```python
from build123d import *

# Parameters (mm, degrees)
F1_DEPTH  = 55
F3_DEPTH  = 50
F4_W      = 46.6654431075
F4_H      = 57.836631313
F5_DEPTH  = 25
F6_R      = 5
F8_D      = 5
F10_DEPTH = 5
F12_DEPTH = 2


with BuildPart() as f1:
    # F0 (on Top) → F1 (new body)
    with BuildSketch(Plane.XY):
        with BuildLine():
            ThreePointArc((0, -20.5), (14.4956890143, -14.4956890143), (20.5, 0))
            ThreePointArc((20.5, 0), (14.4956890143, 14.4956890143), (0, 20.5))
            ThreePointArc((0, 20.5), (-20.5, 0), (0, -20.5))
        make_face()
        with BuildLine():
            ThreePointArc((19, 0), (-13.4350288425, -13.4350288425), (0, 19))
            ThreePointArc((0, 19), (13.4350288425, 13.4350288425), (19, 0))
        make_face(mode=Mode.SUBTRACT)
        with BuildLine():
            ThreePointArc((0, -20.5), (-20.5, 0), (0, 20.5))
            Line((0, 20.5), (-70, 20.5))
            Line((-70, 20.5), (-90, -20.5))
            Line((-90, -20.5), (0, -20.5))
        make_face()
    extrude(amount=F1_DEPTH)

    # F2 (on face) → F3 (cut)
    with BuildSketch(Plane.XY):
        Polygon((-20.693905686, 24.13287099), (-92.3021333856, 24.13287099), (-92.6832251204, -12.49999901), (-75, -15.5), (-75, -22.0035649836), (-20.7452352142, -22.0035649836), align=None)
    extrude(amount=F3_DEPTH, mode=Mode.SUBTRACT)

    # F4 (on face) → F5 (cut)
    with BuildSketch(Plane.XY):
        with Locations((-0.7558101788, 1.7380928621)):
            Rectangle(F4_W, F4_H)
    extrude(amount=F5_DEPTH, mode=Mode.SUBTRACT)

    # F6
    f6_edges = [f1.edges().sort_by_distance(p)[0] for p in [
        (-20.697947, 20.5, 37.5),
        (-20.743562, -20.5, 37.5),
    ]]
    fillet(f6_edges, radius=F6_R)

    # F8 (through all)
    with Locations(Plane.XZ.offset(20.5)):
        with Locations((-80.5, 41.5), (-80.5, 11.5)):
            Hole(F8_D / 2)

    # F9 (on face) → F10 (join)
    with BuildSketch(Plane.XZ.offset(20.5)):
        Polygon((-66.2546011695, 50), (-75, 41.8011878794), (-75, 36.4798588918), (-60.5785174124, 50), align=None)
    extrude(amount=-F10_DEPTH)

    # F11 (on face) → F12 (join)
    with BuildSketch(Plane(origin=(-64.6227775108, 31.5233061028, 0), x_dir=(-0.438423632, -0.8987684456, 0), z_dir=(-0.8987684456, 0.438423632, 0))):
        Polygon((50.1299122344, 50), (38.5309847388, 50), (50.1299122344, 38.7167511187), align=None)
    extrude(amount=-F12_DEPTH)


solid = f1.part
```
Here's how the part is built. I have some questions about the finished solid (model axes, mm). A direction names the side the tool comes from. Give positions to 0.01 mm unless a question says otherwise; leave off trailing zeros. Loops run counter-clockwise (first coordinate to the right, second up) from the corner with the lowest first, then second, coordinate; pieces in that order, holes last. Notation, with made-up numbers: (-8, 43.5) -> (-3, 43.5) arc R6 ccw to (-3, 53.5) -> close; hole circle Ø3 at (66, 34). An arc over 180 degrees is marked (long way). Use one line per item in the form item = value. Start each with the question number.
1) Thinking about a two-plate mould opening in X: for faces 1 (the face through (-69, -15.5, 45)), 2 (the face through (-14, 20.5, 43)), 3 (the face through (-80.9, -14.5, 24.6)), 4 (the face through (-86.62, -13.57, 39.85)), which applies, +X half, -X half, draft (parallel to the pull), parting line (faces both ways), or undercut?
2) Imagine slicing it at C-C (z = 11.5). Please give me the cut outline in (x, y).
3) For P1, Ø4, axis at x = -80.5, z = 11.5, coming from the +Y side; P2, Ø12, axis at y = 5, z = 35, coming from the +X side; P3, Ø1.5, axis at y = -17.5, z = 18, coming from the +X side; P4, Ø11, axis at x = -66, z = 43.5, coming from the +Y side, each with a flat end and sliding along its axis, tell me the tip position at first contact or that it passes through.
4) Imagine slicing it at A-A (z = 32). Please give me the cut outline in (x, y).
5) Imagine slicing it at B-B (y = 14). Please give me the cut outline in (x, z).
6) Which directions (+Z, -Z, +X, -X, +Y, -Y) give clear straight access to the entire face, cutting with the end or side of a thin tool? Please do faces 5 (the face through (-70.566, -18.035, 45.958)), 6 (the face through (-75, -18, 18)), 7 (the face through (-83.17, -11.06, 47.1)), 8 (the face through (-19, 5, 25)), 9 (the face through (-83.137, -8.679, 44.437)).
7) Please list where these lines run through material, in increasing order: line 1 along Z through (x, y) = (-80.5, -18.5); line 2 along Z through (x, y) = (-80, -18); line 3 along X through (y, z) = (-17, 41).
8) Imagine slicing it at D-D (x = -48). Please give me the cut outline in (y, z), then the cut area to 3 significant figures.
Check values:
q1.face_1 = undercut
q1.face_2 = draft
q1.face_3 = undercut
q1.face_4 = -X half
q2.outline = (-90, -20.5) -> (-83, -20.5) -> (-83, -14.14) -> (-86.6, -13.53) -> close; (-78, -20.5) -> (-75, -20.5) -> (-75, -15.5) -> (-78, -14.99) -> close
q3.P1 = through
q3.P2 = 20.5
q3.P3 = -75
q3.P4 = -15.5
q4.outline = (-90, -20.5) -> (-75, -20.5) -> (-75, -15.5) -> (-86.6, -13.53) -> close; (-20.74, -15.49) arc R5 ccw to (-15.74, -20.5) -> (0, -20.5) arc R20.5 ccw to (0, 20.5) -> (-15.7, 20.5) arc R5 ccw to (-20.7, 15.51) -> close; hole circle Ø38 at (0, 0)
q5.outline = (-73.17, 50) -> (-20.71, 50) -> (-20.71, 25) -> (-12.85, 25) -> (-12.85, 55) -> (-73.17, 55) -> close; (12.85, 25) -> (14.97, 25) -> (14.97, 55) -> (12.85, 55) -> close
q6.face_5 = +Y, -Y
q6.face_6 = -Z, +Y, -Y
q6.face_7 = -Z
q6.face_8 = -Z, +X, +Y, -Y
q6.face_9 = -Z, +Y
q7.line_1 = 0 to 9, 14 to 39, 44 to 55
q7.line_2 = 0 to 9.05, 13.95 to 39.05, 43.95 to 55
q7.line_3 = -88.29 to -82.95, -78.05 to -70.18, -20.51 to -8.49, 8.49 to 11.46
q8.outline = (-20.5, 50) -> (20.5, 50) -> (20.5, 55) -> (-20.5, 55) -> close
q8.area = 205 mm^2
